```python
from build123d import *

# Parameters (mm, degrees)
F0_R     = 171.45
F0_R_2   = 7.9375
F0_R_3   = 69.85
F1_DEPTH = 25.4


# Not quite as in the source:
# - ends of sketch curves that miss each other by under 0.0002 mm in the source are joined


with BuildPart() as f1:
    # F0 (on Front) → F1 (new body)
    with BuildSketch(Plane.XZ):
        with Locations((-406.4, 317.5)):
            Circle(F0_R)
        with Locations((-513.8380376, 210.0619624)):
            Circle(F0_R_2, mode=Mode.SUBTRACT)
        with BuildLine():
            Line((-488.75442, 221.659196), (-473.7808914, 239.0848152))
            ThreePointArc((-473.7808914, 239.0848152), (-449.2625045681, 243.2599470835), (-440.6191192625, 219.9388323398))
            Line((-440.6191192625, 219.9388323398), (-448.2233606, 198.2585824))
            ThreePointArc((-448.2233606, 198.2585824), (-482.5999974139, 185.5177169793), (-488.75442, 221.659196))
        make_face(mode=Mode.SUBTRACT)
        with Locations((-553.1630796, 278.174958)):
            Circle(F0_R_2, mode=Mode.SUBTRACT)
        with BuildLine():
            Line((-525.6414176, 275.6766394), (-503.9611714, 283.2808914))
            ThreePointArc((-503.9611714, 283.2808914), (-480.6400529165, 274.6374954319), (-484.8151954053, 250.119120942))
            Line((-484.8151954053, 250.119120942), (-502.240804, 235.14558))
            ThreePointArc((-502.240804, 235.14558), (-538.3822830207, 241.3000025861), (-525.6414176, 275.6766394))
        make_face(mode=Mode.SUBTRACT)
        with Locations((-445.725042, 170.7369204)):
            Circle(F0_R_2, mode=Mode.SUBTRACT)
        with BuildLine():
            Line((-429.800639, 193.3222194), (-425.5459612, 215.9))
            ThreePointArc((-425.5459612, 215.9), (-406.4, 231.775), (-387.2540391788, 215.8999999286))
            Line((-387.2540391788, 215.8999999286), (-382.999361, 193.3222194))
            ThreePointArc((-382.999361, 193.3222194), (-406.4, 165.1), (-429.800639, 193.3222194))
        make_face(mode=Mode.SUBTRACT)
        with Locations((-367.074958, 170.7369204)):
            Circle(F0_R_2, mode=Mode.SUBTRACT)
        with BuildLine():
            Line((-364.5766394, 198.2585824), (-372.1808914, 219.9388286))
            ThreePointArc((-372.1808914, 219.9388286), (-363.5374954319, 243.2599470835), (-339.019120942, 239.0848045947))
            Line((-339.019120942, 239.0848045947), (-324.04558, 221.659196))
            ThreePointArc((-324.04558, 221.659196), (-330.2000025861, 185.5177169793), (-364.5766394, 198.2585824))
        make_face(mode=Mode.SUBTRACT)
        with Locations((-298.9619624, 210.0619624)):
            Circle(F0_R_2, mode=Mode.SUBTRACT)
        with BuildLine():
            Line((-310.559196, 235.14558), (-327.9848152, 250.1191086))
            ThreePointArc((-327.9848152, 250.1191086), (-332.1599470835, 274.6374954319), (-308.8388323398, 283.2808807375))
            Line((-308.8388323398, 283.2808807375), (-287.1585824, 275.6766394))
            ThreePointArc((-287.1585824, 275.6766394), (-274.4177169793, 241.3000025861), (-310.559196, 235.14558))
        make_face(mode=Mode.SUBTRACT)
        with Locations((-259.6369204, 278.174958)):
            Circle(F0_R_2, mode=Mode.SUBTRACT)
        with Locations((-553.1630796, 356.825042)):
            Circle(F0_R_2, mode=Mode.SUBTRACT)
        with BuildLine():
            Line((-530.5777806, 340.900639), (-508, 336.6459612))
            ThreePointArc((-508, 336.6459612), (-492.125, 317.5), (-508.0000000714, 298.3540391788))
            Line((-508.0000000714, 298.3540391788), (-530.5777806, 294.099361))
            ThreePointArc((-530.5777806, 294.099361), (-558.8, 317.5), (-530.5777806, 340.900639))
        make_face(mode=Mode.SUBTRACT)
        with BuildLine():
            Line((-502.240804, 399.85442), (-484.8151848, 384.8808914))
            ThreePointArc((-484.8151848, 384.8808914), (-480.6400529165, 360.3625045681), (-503.9611676602, 351.7191192625))
            Line((-503.9611676602, 351.7191192625), (-525.6414176, 359.3233606))
            ThreePointArc((-525.6414176, 359.3233606), (-538.3822830207, 393.6999974139), (-502.240804, 399.85442))
        make_face(mode=Mode.SUBTRACT)
        with Locations((-513.8380376, 424.9380376)):
            Circle(F0_R_2, mode=Mode.SUBTRACT)
        with BuildLine():
            Line((-448.2233606, 436.7414176), (-440.6191086, 415.0611714))
            ThreePointArc((-440.6191086, 415.0611714), (-449.2625045681, 391.7400529165), (-473.780879058, 395.9151954053))
            Line((-473.780879058, 395.9151954053), (-488.75442, 413.340804))
            ThreePointArc((-488.75442, 413.340804), (-482.5999974139, 449.4822830207), (-448.2233606, 436.7414176))
        make_face(mode=Mode.SUBTRACT)
        with Locations((-406.4, 317.5)):
            Circle(F0_R_3, mode=Mode.SUBTRACT)
        with BuildLine():
            Line((-382.999361, 441.6777806), (-387.2540388, 419.1))
            ThreePointArc((-387.2540388, 419.1), (-406.4, 403.225), (-425.5459608212, 419.1000000714))
            Line((-425.5459608212, 419.1000000714), (-429.800639, 441.6777806))
            ThreePointArc((-429.800639, 441.6777806), (-406.4, 469.9), (-382.999361, 441.6777806))
        make_face(mode=Mode.SUBTRACT)
        with BuildLine():
            Line((-324.04558, 413.340804), (-339.0191086, 395.9151848))
            ThreePointArc((-339.0191086, 395.9151848), (-363.5374954319, 391.7400529165), (-372.1808807375, 415.0611676602))
            Line((-372.1808807375, 415.0611676602), (-364.5766394, 436.7414176))
            ThreePointArc((-364.5766394, 436.7414176), (-330.2000025861, 449.4822830207), (-324.04558, 413.340804))
        make_face(mode=Mode.SUBTRACT)
        with Locations((-445.725042, 464.2630796)):
            Circle(F0_R_2, mode=Mode.SUBTRACT)
        with Locations((-367.074958, 464.2630796)):
            Circle(F0_R_2, mode=Mode.SUBTRACT)
        with BuildLine():
            Line((-282.2222194, 294.099361), (-304.8, 298.3540388))
            ThreePointArc((-304.8, 298.3540388), (-320.675, 317.5), (-304.7999999286, 336.6459608212))
            Line((-304.7999999286, 336.6459608212), (-282.2222194, 340.900639))
            ThreePointArc((-282.2222194, 340.900639), (-254, 317.5), (-282.2222194, 294.099361))
        make_face(mode=Mode.SUBTRACT)
        with BuildLine():
            Line((-287.1585824, 359.3233606), (-308.8388286, 351.7191086))
            ThreePointArc((-308.8388286, 351.7191086), (-332.1599470835, 360.3625045681), (-327.9848045947, 384.880879058))
            Line((-327.9848045947, 384.880879058), (-310.559196, 399.85442))
            ThreePointArc((-310.559196, 399.85442), (-274.4177169793, 393.6999974139), (-287.1585824, 359.3233606))
        make_face(mode=Mode.SUBTRACT)
        with Locations((-259.6369204, 356.825042)):
            Circle(F0_R_2, mode=Mode.SUBTRACT)
        with Locations((-298.9619624, 424.9380376)):
            Circle(F0_R_2, mode=Mode.SUBTRACT)
    extrude(amount=F1_DEPTH)


solid = f1.part
```
Geometry check sheet. Reference: the model listing, model coordinates, mm. Coordinates: 2 decimals unless noted, no trailing zeros. Loops run counter-clockwise (first coordinate to the right, second up) from the corner with the lowest first, then second, coordinate; pieces in that order, holes last. Notation, with made-up numbers: (70.5, -2.5) - (103.5, -2.5) arc R18 ccw to (103.5, 4.5) - close; hole circle Ø2 at (87, 46.25). An arc over 180 degrees is marked (long way). One line per item, written item: value. Start each with the question number.
(1) Cross-section at B-B on x = -412. Enter the section's corners in (y, z).
(2) Depth check by flat-ended pin: P1, Ø3, axis at y = -22.5, z = 196.5, coming from the -X side; P2, Ø12.5, axis at x = -367.07, z = 170.74, coming from the +Y side; P3, Ø1.5, axis at y = -15, z = 296.5, coming from the +X side; P4, Ø18.5, axis at x = -259.64, z = 278.17, coming from the +Y side. Enter the tip coordinate at first touch or a pass-through.
(3) Cross-section at A-A on z = 317.5. Enter the section's corners in (x, y) (3 decimals), plus the area to 3 significant figures.
(4) Mould release check, pull along Z, two halves, no side actions. Record for faces 1 (the cylindrical face through (-320.67, -12.52, 317.12)), 2 (the cylindrical face through (-428.72, -12.52, 487.49)): released by +Z, released by -Z, zero draft, split by the parting line, or undercut.
(5) Cross-section at C-C on y = -20.75. Count the separate pieces of the cut face and the enclosed holes in it, plus the area to 3 significant figures.
(6) Material ranges on line 1 (Z direction, x = -487, y = -2.75); line 2 (X direction, y = -8.5, z = 332); line 3 (X direction, y = -22.5, z = 447.5), recorded low to high. Write a range as [from, to].
Results below:
1. outline: (-25.4, 146.14) - (0, 146.14) - (0, 165.77) - (-25.4, 165.77) - close; (-25.4, 230.95) - (0, 230.95) - (0, 247.87) - (-25.4, 247.87) - close; (-25.4, 387.13) - (0, 387.13) - (0, 404.05) - (-25.4, 404.05) - close; (-25.4, 469.23) - (0, 469.23) - (0, 488.86) - (-25.4, 488.86) - close
2. P1: stops at x = -529.34
2. P2: passes through
2. P3: stops at x = -236.15
2. P4: stops at y = 0
3. outline: (-577.85, -25.4) - (-558.8, -25.4) - (-558.8, 0) - (-577.85, 0) - close; (-492.125, -25.4) - (-476.25, -25.4) - (-476.25, 0) - (-492.125, 0) - close; (-336.55, -25.4) - (-320.675, -25.4) - (-320.675, 0) - (-336.55, 0) - close; (-254, -25.4) - (-234.95, -25.4) - (-234.95, 0) - (-254, 0) - close
3. area: 1,770 mm2
4. face 1: undercut
4. face 2: split by the parting line
5. separate pieces: 1
5. enclosed holes: 25
5. area: 44,400 mm2
6. line 1: z = [166.18, 188.79], [223.7, 248.24], [281.3, 353.7], [386.76, 411.3], [446.21, 468.82]
6. line 2: x = [-577.24, -553.88], [-498.6, -474.73], [-338.07, -314.2], [-258.92, -235.56]
6. line 3: x = [-518.18, -485.51], [-455.88, -430.17], [-382.63, -356.92], [-327.29, -294.62]
